Verification items for this drawing (mm, ordinates from the low corner). Coordinates: 2 decimals unless noted, no trailing zeros. Write each loop counter-clockwise with the first axis right and the second up, starting at its lowest first coordinate (ties: lowest second). Pieces come first, ordered by that corner, then holes.
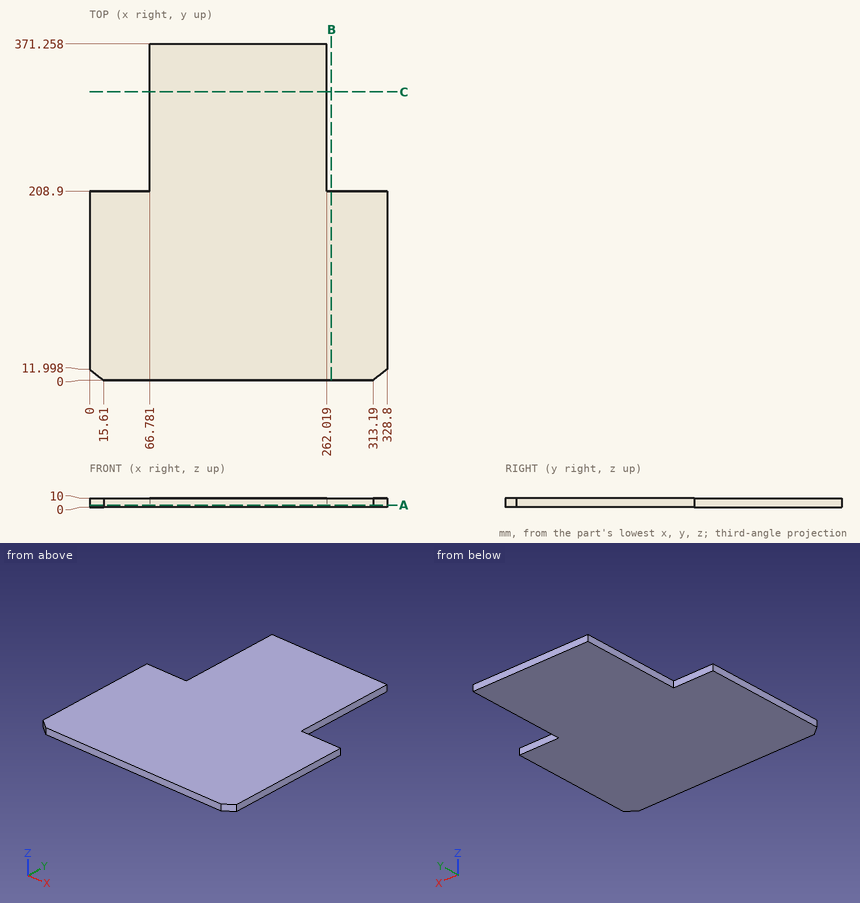
1. Thickness scan on line 1 along Y through (x, z) = (287, 3); line 2 along X through (y, z) = (252, 8). Record the ranges inside material, lowest first.
Computed values:
line 1: y = 0 to 208.9
line 2: x = 66.78 to 262.02
2. Gauge pin test, flat ends, axial feed: pin 1 Ø5 at (x, z) = (283.5, 3) entering from +Y; pin 2 Ø3 at (y, z) = (296.5, 7) entering from +X. Record the tip position at first contact, or that the pin passes through.
Computed values:
pin 1: stops at y = 208.9
pin 2: stops at x = 262.02
3. Sectioned sample at B-B, the plane x = 267. Record the boundary of the cut face in (y, z).
Computed values:
outline: (0, 0) - (208.9, 0) - (208.9, 10) - (0, 10) - close
4. Sectioned sample at C-C, the plane y = 318.5. Record the boundary of the cut face in (x, z), and give its area (3 significant figures).
Computed values:
outline: (66.78, 0) - (262.02, 0) - (262.02, 10) - (66.78, 10) - close
area: 1,950 mm2
5. Sectioned sample at A-A, the plane z = 2.5. Record the boundary of the cut face in (x, y).
Computed values:
outline: (0, 12) - (15.61, 0) - (313.19, 0) - (328.8, 12) - (328.8, 208.9) - (262.02, 208.9) - (262.02, 371.26) - (66.78, 371.26) - (66.78, 208.9) - (0, 208.9) - close
